Study the drawing (mm; zero at the part's minimum x, y, z) and answer. A direction names the side the tool comes from. Coordinates: 2 decimals unless noted, no trailing zeros. Order: outer loops, then holes, each group sorted by start corner. A loop starts at its lowest first (then second) coordinate and runs counter-clockwise, first axis right, second up. Notation, with made-up numbers: M 89,-26 L 104,-26 A18 cw 104,8 Z; hole C -10.75,41 d10. An arc over 180 degrees is marked long. Put each result on its own line as item: value.
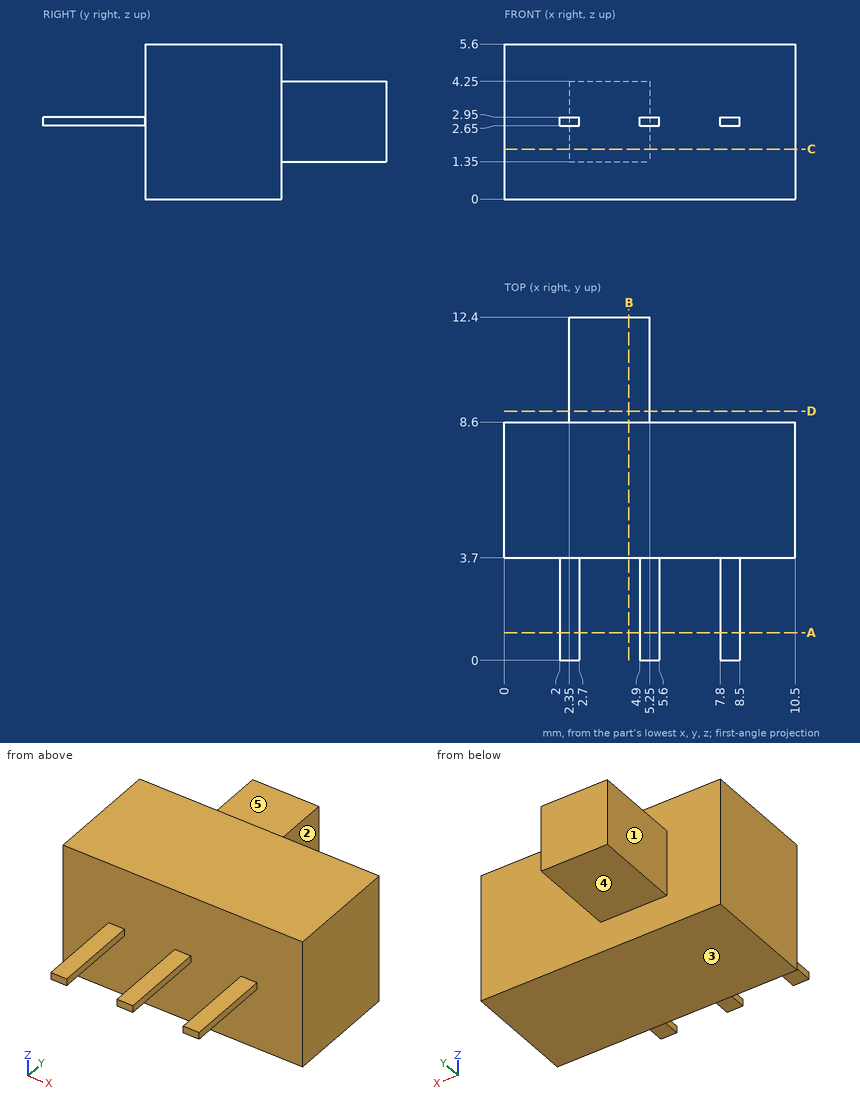
Q1. Find section A-A on y = 1. Write down the section's boundary in (x, z).
Answers below:
outline: M 2,2.65 L 2.7,2.65 L 2.7,2.95 L 2,2.95 Z; M 4.9,2.65 L 5.6,2.65 L 5.6,2.95 L 4.9,2.95 Z; M 7.8,2.65 L 8.5,2.65 L 8.5,2.95 L 7.8,2.95 Z
Q2. Find section C-C on z = 1.8. Write down the section's boundary in (x, y), plus the area to 3 significant figures.
Answers below:
outline: M 0,3.7 L 10.5,3.7 L 10.5,8.6 L 5.25,8.6 L 5.25,12.4 L 2.35,12.4 L 2.35,8.6 L 0,8.6 Z
area: 62.5 mm^2
Q3. Given pin 1 (0.6 mm diameter, centred on x = 5.5, y = 2.5, fed in from +Z); pin 2 (0.6 mm diameter, centred on x = 5, y = 2.5, fed in from -Z); pin 3 (3 mm diameter, centred on y = 11, z = 3, fed in from +X), each flat-ended and moving along its own axis, determine where each tip first touches the part or whether it passes through.
Answers below:
pin 1: stops at z = 2.95
pin 2: stops at z = 2.65
pin 3: stops at x = 5.25
Q4. A tool of negligible diameter and unlimited length cuts with its end or side. For the marked faces 1, 2, 3, 4 and 5, from which of +Z, -Z, +X, -X, +Y, -Y can it reach the whole face along a straight path? Write none if from no direction.
Answers below:
face 1: +Z, -Z, -X, +Y
face 2: +Z, -Z, +X, +Y
face 3: -Z, +X, -X, +Y, -Y
face 4: -Z, +X, -X, +Y
face 5: +Z, +X, -X, +Y
Q5. Find section D-D on y = 9. Write down the section's boundary in (x, z).
Answers below:
outline: M 2.35,1.35 L 5.25,1.35 L 5.25,4.25 L 2.35,4.25 Z
Q6. Consider line 1 along Y through (x, z) = (6, 1.9); line 2 along Z through (x, y) = (4, 8.75); line 3 along X through (y, z) = (11.5, 3.7). Determine where each line is inside the solid, lowest interval first.
Answers below:
line 1: y = 3.7 to 8.6
line 2: z = 1.35 to 4.25
line 3: x = 2.35 to 5.25
Q7. Find section B-B on x = 4.5. Write down the section's boundary in (y, z).
Answers below:
outline: M 3.7,0 L 8.6,0 L 8.6,1.35 L 12.4,1.35 L 12.4,4.25 L 8.6,4.25 L 8.6,5.6 L 3.7,5.6 Z
